Could you check a few things on this model? Use its own coordinates, in mm. Face numbers are marked on the shaded views. A direction names the side the tool comes from. Give positions to 0.01 mm unless a question says otherwise; leave off trailing zeros. Order: outer loops, then holes, each group sorted by start corner. A loop starts at its lowest first (then second) coordinate and runs counter-clockwise, first axis right, second up. Notation, with made-up numbers: M 77,65 L 118,65 A18 ccw 118,89 Z; hole C 72,-7.75 d7. An arc over 180 degrees is marked long. Answer in a Markdown table with one row per item. Add a question column.
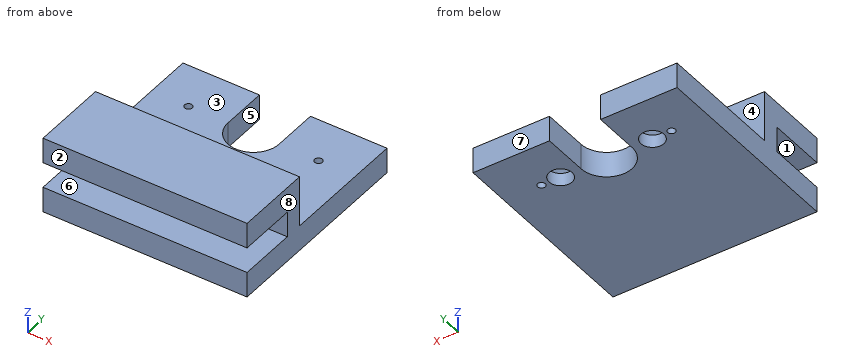
```python
from build123d import *

# Parameters (mm, degrees)
F1_DEPTH = 10
F2_W     = 80
F2_H     = 7
F3_DEPTH = 20
F4_W     = 80
F4_H     = 10
F5_DEPTH = 23
F6_D     = 3
F7_D     = 3
F8_D     = 9
F8_DEPTH = 5
F8_TIP   = 2.7038727856


with BuildPart() as f1:
    # F0 (on Top) → F1 (new body)
    with BuildSketch(Plane.XY):
        with BuildLine():
            Line((-40, -40), (40, -40))
            Line((40, -40), (40, 40))
            Line((40, 40), (10, 40))
            Line((10, 40), (10, 22))
            ThreePointArc((10, 22), (0, 12), (-10, 22))
            Line((-10, 22), (-10, 40))
            Line((-10, 40), (-40, 40))
            Line((-40, 40), (-40, -40))
        make_face()
    extrude(amount=F1_DEPTH)

    # F2 (on face) → F3 (join)
    with BuildSketch(Plane.XY.offset(10)):
        with Locations((0, -13.5)):
            Rectangle(F2_W, F2_H)
    extrude(amount=F3_DEPTH)

    # F4 (on face) → F5 (join)
    with BuildSketch(Plane.XZ.offset(17)):
        with Locations((0, 25)):
            Rectangle(F4_W, F4_H)
    extrude(amount=F5_DEPTH)

    # F6 (through all)
    with Locations(Plane(origin=(0, 0, 0), x_dir=(1, 0, 0), z_dir=(0, 0, -1))):
        with Locations((25.5, -22)):
            Hole(F6_D / 2)

    # F7 (through all)
    with Locations(Plane(origin=(0, 0, 0), x_dir=(1, 0, 0), z_dir=(0, 0, -1))):
        with Locations((-25.5, -22)):
            Hole(F7_D / 2)

    # F8
    with Locations(Plane(origin=(0, 0, 0), x_dir=(1, 0, 0), z_dir=(0, 0, -1))):
        with Locations((18, -22), (-18, -22)):
            Hole(F8_D / 2, depth=F8_DEPTH)
            with Locations((0, 0, -(F8_DEPTH + F8_TIP / 2))):  # 118° drill point
                Cone(0, F8_D / 2, F8_TIP, mode=Mode.SUBTRACT)


solid = f1.part
```
1. For the marked faces 4, 5, 6, 7 and 8, which set-ups out of +Z, -Z, +X, -X, +Y, -Y let a thin tool reach every point of the face, with its end or its side?
2. Thinking about a two-plate mould opening in Z: for the marked faces 1, 2 and 3, which applies, pulls with the +Z half, pulls with the -Z half, needs draft (parallel to the pull), parting line crosses it, or undercut?
3. Will these pins go through, and if not, where does the flat tip stop? P1, Ø1, axis at x = 0.5, z = 15, coming from the +Y side; P2, Ø4, axis at x = -25.5, y = 22, coming from the +Z side; P3, Ø3, axis at x = 13, z = 15, coming from the -Y side.
4. Suppose I cut it at C-C on x = 0. List the corners of the cut face in (y, z) for me, plus the area to 3 significant figures.
5. If I drill on line 1 along X through (y, z) = (22, 4.5); line 2 along Y through (x, z) = (-25.5, 7.5); line 3 along X through (y, z) = (24, 7.75), over which ranges is the centre line in solid material (lowest first)? Write a range as [from, to].
6. Suppose I cut it at D-D on z = 18.25. List the corners of the cut face in (x, y) for me, plus the area to 3 significant figures.
7. Suppose I cut it at A-A on x = 25.5. List the corners of the cut face in (y, z) for me.
8. Suppose I cut it at B-B on z = 9. List the corners of the cut face in (x, y) for me.
Findings below:
| question | item | result |
|---|---|---|
| 1 | face 4 | +Z, +X, -X, +Y |
| 1 | face 5 | +Z, -Z, +Y |
| 1 | face 6 | +X, -X, -Y |
| 1 | face 7 | +Z, -Z, +X, -X, +Y |
| 1 | face 8 | +Z, -Z, +X, +Y, -Y |
| 2 | face 1 | undercut |
| 2 | face 2 | needs draft |
| 2 | face 3 | pulls with the +Z half |
| 3 | P1 | y = -10 |
| 3 | P2 | z = 10 |
| 3 | P3 | y = -17 |
| 4 | outline | M -40,0 L 12,0 L 12,10 L -10,10 L -10,30 L -40,30 L -40,20 L -17,20 L -17,10 L -40,10 Z |
| 4 | area | 890 mm2 |
| 5 | line 1 | [-40, -27], [-24, -22.5], [-13.5, -10], [10, 13.5], [22.5, 24], [27, 40] |
| 5 | line 2 | [-40, 20.5], [23.5, 40] |
| 5 | line 3 | [-40, -10], [10, 40] |
| 6 | outline | M -40,-17 L 40,-17 L 40,-10 L -40,-10 Z |
| 6 | area | 560 mm2 |
| 7 | outline | M -40,0 L 20.5,0 L 20.5,10 L -10,10 L -10,30 L -40,30 L -40,20 L -17,20 L -17,10 L -40,10 Z; M 23.5,0 L 40,0 L 40,10 L 23.5,10 Z |
| 8 | outline | M -40,-40 L 40,-40 L 40,40 L 10,40 L 10,22 A10 cw -10,22 L -10,40 L -40,40 Z; hole C -25.5,22 d3; hole C 25.5,22 d3 |
